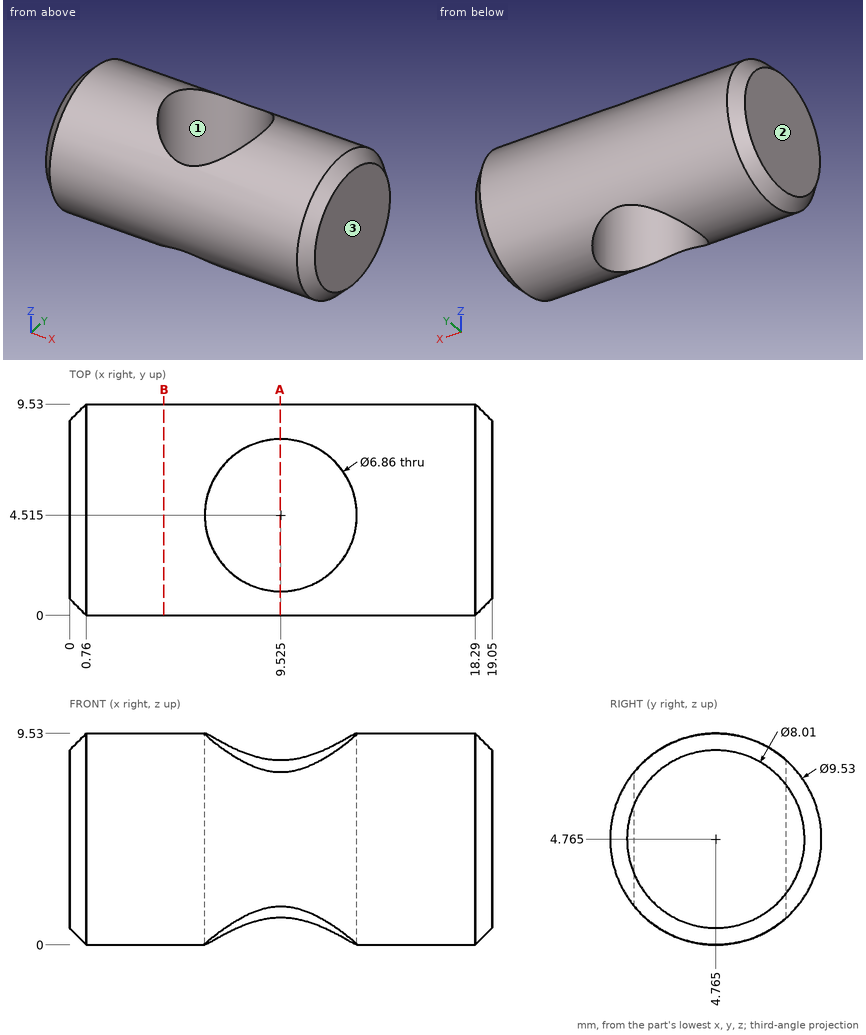
Could you check a few things on this drawing? It's one solid part, dimensions in mm from its lowest x, y, z. Coordinates: 2 decimals unless noted, no trailing zeros. Order: outer loops, then holes, each group sorted by start corner. A loop starts at its lowest first (then second) coordinate and runs counter-clockwise, first axis right, second up. Notation, with made-up numbers: M 14,-38 L 56,-38 A7 ccw 56,-31 Z; hole C 22,-8 d10. An arc over 180 degrees is marked long. Use one line per item in the form item = value. Start each with the question number.
1. Please list where these lines run through material, in increasing order: line 1 (X direction, y = 4.25, z = 3); line 2 (Y direction, x = 6.5, z = 9); line 3 (Y direction, x = 12.5, z = 8.5).
2. We'd pull the mould along X, two halves only. Please class the marked faces 1, 2 and 3: +X half, -X half, draft (parallel to the pull), parting line (faces both ways), or undercut.
3. Suppose I cut it at B-B on x = 4.25. Write out the boundary of the cut face in (y, z) (3 decimals), then the cut area to 3 significant figures.
4. Suppose I cut it at A-A on x = 9.5. Write out the boundary of the cut face in (y, z) (3 decimals).
5. For pin 1 (2 mm diameter, centred on x = 11.5, y = 8.5, fed in from -Z); pin 2 (1.5 mm diameter, centred on x = 11.5, y = 1, fed in from -Z), each with a flat end and sliding along its axis, tell me the tip position at first contact or that it passes through.
Geometry says:
q1.line_1 = 0 to 6.11, 12.94 to 19.05
q1.line_2 = 2.58 to 2.9, 6.13 to 6.95
q1.line_3 = 1.81 to 2.81, 6.22 to 7.72
q2.face_1 = undercut
q2.face_2 = -X half
q2.face_3 = +X half
q3.outline = C 4.765,4.765 d9.53
q3.area = 71.3 mm^2
q4.outline = M 1.085,1.738 L 1.085,7.792 A4.765 ccw Z; M 7.945,1.216 A4.765 ccw 7.945,8.314 Z
q5.pin_1 = 0.86
q5.pin_2 = 1.08
